from build123d import *

# Parameters (mm, degrees)
F0_W     = 104.775
F0_H     = 117.475
F0_W_2   = 92.075
F0_H_2   = 104.775
F1_DEPTH = 69.85
F2_W     = 104.775
F2_H     = 117.475
F2_W_2   = 92.075
F2_H_2   = 104.775
F3_DEPTH = 6.35


with BuildPart() as f1:
    # F0 (on Top) → F1 (new body)
    with BuildSketch(Plane.XY):
        with Locations((52.3875, 58.7375)):
            Rectangle(F0_W, F0_H)
        with Locations((52.3875, 58.7375)):
            Rectangle(F0_W_2, F0_H_2, mode=Mode.SUBTRACT)
    extrude(amount=F1_DEPTH)

    # F2 (on face) → F3 (join)
    with BuildSketch(Plane.XY.offset(69.85)):
        with Locations((52.3875, 58.7375)):
            Rectangle(F2_W, F2_H)
        with Locations((52.3875, 58.7375)):
            Rectangle(F2_W_2, F2_H_2, mode=Mode.SUBTRACT)
        with Locations((52.3875, 58.7375)):
            Rectangle(F2_W_2, F2_H_2)
    extrude(amount=F3_DEPTH)


solid = f1.part
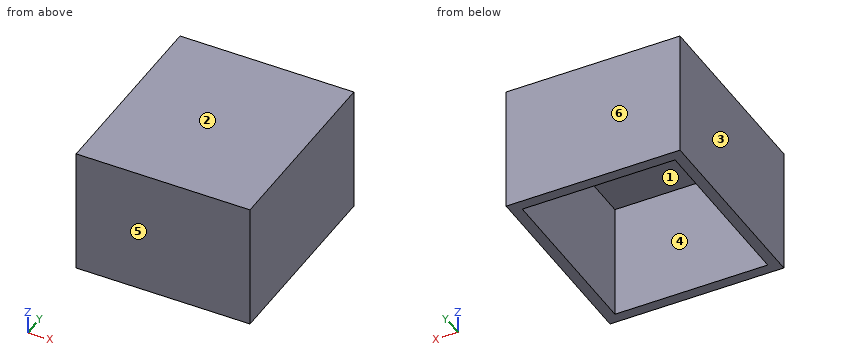
Geometry check sheet. Reference: the model listing, model coordinates, mm. Face numbers are marked on the shaded views. A direction names the side the tool comes from. Give positions to 0.01 mm unless a question says otherwise; leave off trailing zeros. Write each loop counter-clockwise with the first axis right and the second up, starting at its lowest first coordinate (ties: lowest second). Pieces come first, ordered by that corner, then holes. Notation, with made-up numbers: M -26,-1.75 L 21,-1.75 A14 ccw 21,5.25 Z; hole C 44,26 d2. An arc over 180 degrees is marked long. One line per question, with ' | ' between items.
1. Scan lines: line 1 along Y through (x, z) = (19.5, 66.5) (3 decimals); line 2 along X through (y, z) = (7, 14) (3 decimals); line 3 along Z through (x, y) = (56.5, 68). Record each from-to range of solid material in increasing order. Write a range as from..to.
Ans:
line 1: 0..6.35, 111.125..117.475 | line 2: 0..6.35, 98.425..104.775 | line 3: 69.85..76.2
2. Cross-section at C-C (x = 89.5). Enter the section's corners in (y, z) (3 decimals), plus the area to 3 significant figures.
Ans:
outline: M 0,0 L 6.35,0 L 6.35,69.85 L 111.125,69.85 L 111.125,0 L 117.475,0 L 117.475,76.2 L 0,76.2 Z | area: 1,630 mm2
3. Cross-section at A-A (z = 46). Enter the section's corners in (x, y) (3 decimals), plus the area to 3 significant figures.
Ans:
outline: M 0,0 L 104.775,0 L 104.775,117.475 L 0,117.475 Z; hole M 6.35,6.35 L 98.425,6.35 L 98.425,111.125 L 6.35,111.125 Z | area: 2,660 mm2
4. Gauge pin test, flat ends, axial feed: pin 1 (1 mm diameter, centred on x = 44, z = 33.5, fed in from -Y); pin 2 (4 mm diameter, centred on x = 38.5, y = 84, fed in from -Z). Record the tip position at first contact, or that the pin passes through.
Ans:
pin 1: y = 0 | pin 2: z = 69.85
5. Cross-section at B-B (y = 68.5). Enter the section's corners in (x, z) (3 decimals), plus the area to 3 significant figures.
Ans:
outline: M 0,0 L 6.35,0 L 6.35,69.85 L 98.425,69.85 L 98.425,0 L 104.775,0 L 104.775,76.2 L 0,76.2 Z | area: 1,550 mm2
6. Mould release check, pull along Y, two halves, no side actions. Record for the marked faces 3, 4, 5 and 6: released by +Y, released by -Y, zero draft, split by the parting line, or undercut.
Ans:
face 3: zero draft | face 4: undercut | face 5: released by -Y | face 6: released by +Y
7. Set-up check for the marked faces 1 and 2: record each of +Z, -Z, +X, -X, +Y, -Y from which the full face is reachable in a straight line by a thin tool's end or side.
Ans:
face 1: -Z | face 2: +Z, +X, -X, +Y, -Y
